Geometry check sheet. Reference: the model listing, model coordinates, mm. Round coordinates to 2 decimals unless told otherwise and drop trailing zeros. Write each loop counter-clockwise with the first axis right and the second up, starting at its lowest first coordinate (ties: lowest second). Pieces come first, ordered by that corner, then holes. Notation, with made-up numbers: (-8, -26.5) -> (45, -26.5) arc R33 ccw to (45, 8.5) -> close; hole circle Ø9 at (43.5, 48.5). An arc over 180 degrees is marked (long way). Use a Markdown table: item, result.
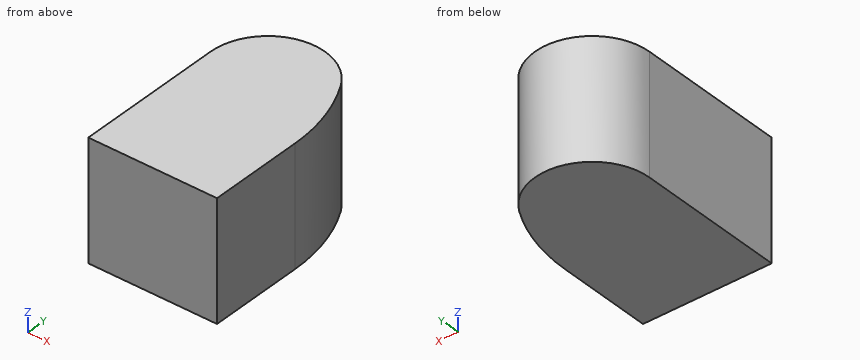
```python
from build123d import *

# Parameters (mm, degrees)
F0_W        = 50.8
F0_H        = 101.6
F1_DEPTH    = 46.99
F2_T1_DEPTH = 366.5870593472
F3_R        = 22.587582604


# Not quite as in the source:
# - a fillet or chamfer that OpenCascade refuses, or shapes differently, is made with other operations: its cross-section is extruded or revolved along the edge and cut away or added


with BuildPart() as f1:
    # F0 (on Top) → F1 (new body)
    with BuildSketch(Plane.XY):
        with Locations((87.8112020218, -9.4523200796)):
            Rectangle(F0_W, F0_H)
    extrude(amount=F1_DEPTH)

    # F2: fillet of radius 65.6134961982 on 1 edges, made by hand

    # F2_s2 → F2_t1 (cut)
    with BuildSketch(Plane.XY.offset(-159.7985296736)):
        with BuildLine():
            ThreePointArc((62.4112020218, 41.3476799204), (98.964505217, 18.2520699738), (113.2112020218, -22.571731949))
            Line((113.2112020218, -22.571731949), (113.2112020218, 41.3476799204))
            Line((113.2112020218, 41.3476799204), (62.4112020218, 41.3476799204))
        make_face()
    extrude(amount=F2_T1_DEPTH, mode=Mode.SUBTRACT)

    # F3
    f3_edges = [f1.edges().sort_by_distance(p)[0] for p in [
        (62.411202, 41.34768, 23.495),
    ]]
    fillet(f3_edges, radius=F3_R)


solid = f1.part
```
(1) Section check C-C on y = -11.5. Record the cut outline in (x, z).
A:
| item | result |
|---|---|
| outline | (62.41, 0) -> (112.27, 0) -> (112.27, 46.99) -> (62.41, 46.99) -> close |
(2) Gauge pin test, flat ends, axial feed: pin 1 Ø2 at (x, z) = (70.5, 22) entering from +Y; pin 2 Ø4 at (y, z) = (5, 14) entering from -X; pin 3 Ø10 at (x, y) = (75, -23) entering from -Z; pin 4 Ø1.5 at (x, z) = (71.5, 29.5) entering from +Y. Record the tip position at first contact, or that the pin passes through.
A:
| item | result |
|---|---|
| pin 1 | stops at y = 16.81 |
| pin 2 | stops at x = 62.82 |
| pin 3 | stops at z = 0 |
| pin 4 | stops at y = 17.34 |
(3) Section check A-A on z = 30.5. Record the cut outline in (x, y).
A:
| item | result |
|---|---|
| outline | (62.41, -60.25) -> (113.21, -60.25) -> (113.21, -22.57) arc R65.61 ccw to (104.63, 9.86) arc R22.59 ccw to (62.41, -1.3) -> close |
(4) Thickness scan on line 1 (Y direction, x = 85, z = 18); line 2 (Y direction, x = 80, z = 21); line 3 (X direction, y = 14.5, z = 32). Record the ranges inside material, lowest first.
A:
| item | result |
|---|---|
| line 1 | y = -60.25 to 21.29 |
| line 2 | y = -60.25 to 20.73 |
| line 3 | x = 68.86 to 101.14 |
(5) Section check B-B on x = 75. Record the cut outline in (y, z), plus the area to 3 significant figures.
A:
| item | result |
|---|---|
| outline | (-60.25, 0) -> (18.95, 0) -> (18.95, 46.99) -> (-60.25, 46.99) -> close |
| area | 3,720 mm2 |
